For this review, use the dimensioned drawing (mm, ordinates from the lowest corner) and the shaded views. A direction names the side the tool comes from. Round coordinates to 2 decimals unless told otherwise and drop trailing zeros. Write each loop counter-clockwise with the first axis right and the second up, starting at its lowest first coordinate (ties: lowest second). Pieces come first, ordered by that corner, then holes.
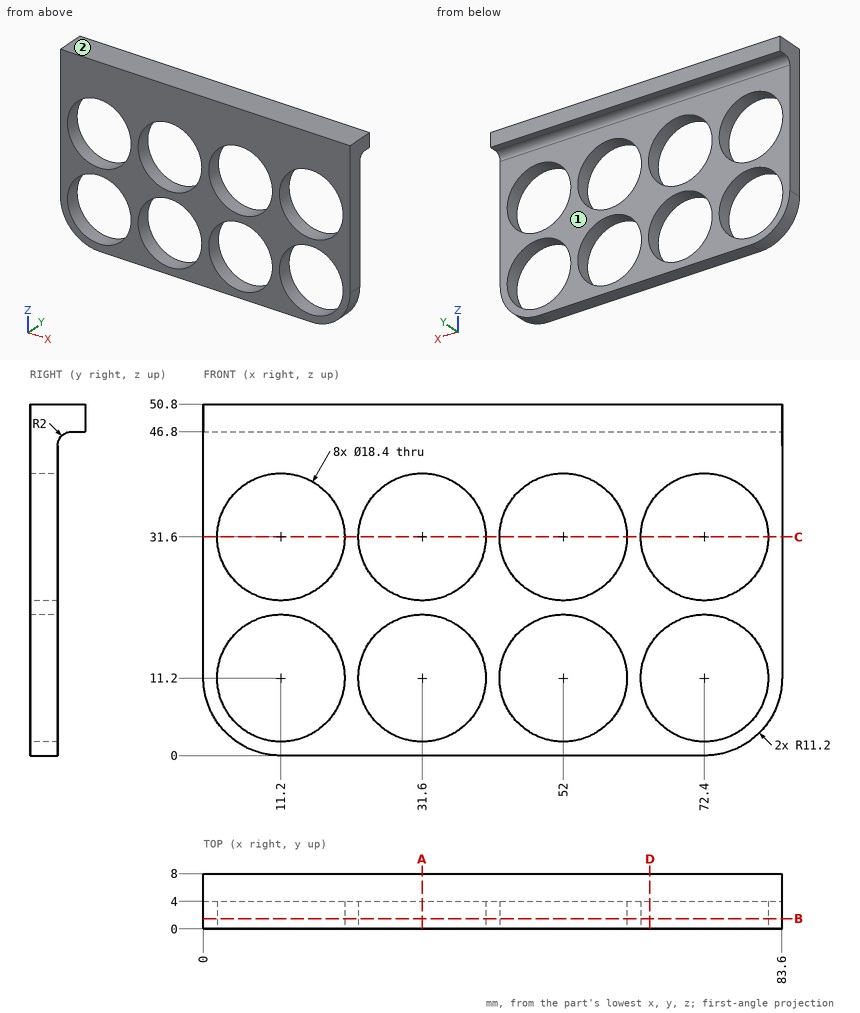
1) Add section A-A on x = 31.6. State the section outline as (y, z) points.
2) Add section C-C on z = 31.6. State the section outline as (x, y) points.
3) For the marked faces 1 and 2, list the 3-axis set-ups (+Z, -Z, +X, -X, +Y, -Y) from which the entire face can be reached by the end or side of a thin tool; tool diameter is ignored.
4) For P1, Ø1.6, axis at x = 36.5, y = 7.5, coming from the -Z side; P2, Ø22.5, axis at x = 47, z = 19.5, coming from the +Y side, all flat-tipped, find the tip position at first contact; note any pin that passes through.
5) Add section D-D on x = 64.5. State the section outline as (y, z) points, and give its area (3 significant figures).
6) Add section B-B on y = 1.5. Count the separate pieces of the cut face and the enclosed holes in it, and give its area (3 significant figures).
7) For line 1 along X through (y, z) = (2.3, 31.6); line 2 along Z through (x, y) = (28.5, 0.5); line 3 along Z through (x, y) = (76.5, 0.5), list the stretches that pass through material, from the lowest coordinate up.
Computed:
1. outline: (0, 0) - (4, 0) - (4, 2) - (0, 2) - close; (0, 20.4) - (4, 20.4) - (4, 22.4) - (0, 22.4) - close; (0, 40.8) - (4, 40.8) - (4, 44.8) arc R2 cw to (6, 46.8) - (8, 46.8) - (8, 50.8) - (0, 50.8) - close
2. outline: (0, 0) - (2, 0) - (2, 4) - (0, 4) - close; (20.4, 0) - (22.4, 0) - (22.4, 4) - (20.4, 4) - close; (40.8, 0) - (42.8, 0) - (42.8, 4) - (40.8, 4) - close; (61.2, 0) - (63.2, 0) - (63.2, 4) - (61.2, 4) - close; (81.6, 0) - (83.6, 0) - (83.6, 4) - (81.6, 4) - close
3. face 1: -Z, +X, -X, +Y
3. face 2: +Z, +X, -X, +Y, -Y
4. P1: stops at z = 46.8
4. P2: stops at y = 4
5. outline: (0, 0) - (4, 0) - (4, 6.49) - (0, 6.49) - close; (0, 15.91) - (4, 15.91) - (4, 26.89) - (0, 26.89) - close; (0, 36.31) - (4, 36.31) - (4, 44.8) arc R2 cw to (6, 46.8) - (8, 46.8) - (8, 50.8) - (0, 50.8) - close
5. area: 145 mm2
6. separate pieces: 1
6. enclosed holes: 8
6. area: 2,070 mm2
7. line 1: x = 0 to 2, 20.4 to 22.4, 40.8 to 42.8, 61.2 to 63.2, 81.6 to 83.6
7. line 2: z = 0 to 2.54, 19.86 to 22.94, 40.26 to 50.8
7. line 3: z = 0.78 to 2.96, 19.44 to 23.36, 39.84 to 50.8
